from build123d import *

# Parameters (mm, degrees)
SKETCH1_R           = 10
SKETCH1_R_2         = 1
BOSS_EXTRUDE1_DEPTH = 4
SKETCH2_R           = 1.75
SKETCH2_R_2         = 1
BOSS_EXTRUDE2_DEPTH = 22
CHAMFER1_SIZE       = 1
SKETCH3_R           = 1
CUT_EXTRUDE1_DEPTH  = 26.943448113


with BuildPart() as part:
    # Sketch1 → Boss-Extrude1 (new body)
    with BuildSketch(Plane.XY):
        Circle(SKETCH1_R)
        Circle(SKETCH1_R_2, mode=Mode.SUBTRACT)
    extrude(amount=BOSS_EXTRUDE1_DEPTH)

    # Sketch2 → Boss-Extrude2 (add)
    with BuildSketch(Plane.XY.offset(4)):
        Circle(SKETCH2_R)
        Circle(SKETCH2_R_2, mode=Mode.SUBTRACT)
    extrude(amount=BOSS_EXTRUDE2_DEPTH)

    # Chamfer1
    # the kernel refuses this chamfer: 1 mm, written as the material it takes off along each edge
    with BuildSketch(Plane(origin=(0, 0, 26), x_dir=(1, 0, 0), z_dir=(0, -1, 0))) as chamfer1_piece_1:
        Polygon((1.75, -CHAMFER1_SIZE), (1.75 - CHAMFER1_SIZE, 0), (1.75, 0), align=None)
    revolve(axis=Axis((0, 0, 26), (0, 0, 1)), mode=Mode.SUBTRACT)

    # Sketch3 → Cut-Extrude1 (cut, through all)
    with BuildSketch(Plane.XY.offset(4)):
        with Locations((0, 7.5)):
            Circle(SKETCH3_R)
        with Locations((-7.5, 0)):
            Circle(SKETCH3_R)
        with Locations((7.5, 0)):
            Circle(SKETCH3_R)
        with Locations((0, -7.5)):
            Circle(SKETCH3_R)
    extrude(amount=-CUT_EXTRUDE1_DEPTH, mode=Mode.SUBTRACT)


solid = part.part
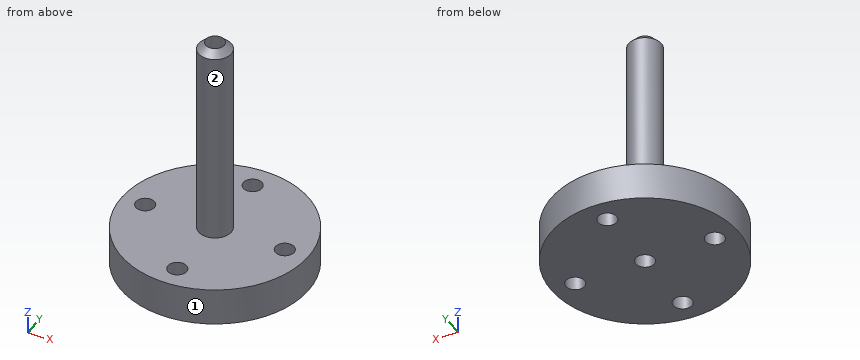
The model under review builds one solid part; all positions refer to its coordinate system, in mm. Face numbers are marked on the shaded views. A direction names the side the tool comes from. Round coordinates to 2 decimals unless told otherwise and drop trailing zeros. Loops run counter-clockwise (first coordinate to the right, second up) from the corner with the lowest first, then second, coordinate; pieces in that order, holes last. Notation, with made-up numbers: M 54,71 L 72,71 A12 cw 72,93 Z; hole C 79.25,19 d7. An arc over 180 degrees is marked long. Answer as CSV lines item,"result". Start each with the question number.
Item 1: For the marked faces 1 and 2, list the 3-axis set-ups (+Z, -Z, +X, -X, +Y, -Y) from which the entire face can be reached by the end or side of a thin tool; tool diameter is ignored.
Item 2: Wall thickness on line 1 (Y direction, x = 0, z = 3.2); line 2 (Y direction, x = 0, z = 14); line 3 (Z direction, x = 0.75, y = 6): over which ranges is each line inside the solid? List them lowest first. Write a range as [from, to].
Item 3: Consider section C-C (y = -7.5). Write out the cut boundary in (x, z), then the cut area to 3 significant figures.
Item 4: Insertion check: P1, Ø1.2, axis at x = 7.5, y = 0, coming from the +Z side; P2, Ø12, axis at x = 2, y = 2.5, coming from the -Z side; P3, Ø3, axis at x = -6, z = 4, coming from the -Y side; P4, Ø6, axis at x = -3, y = -3.5, coming from the +Z side. Each pin has a flat end and moves straight along its axis. Give the tip position at first contact, or say it passes through.
Item 5: Consider section A-A (x = 0). Write out the cut boundary in (y, z).
Answer:
1,face 1,"+Z, -Z"
1,face 2,"+Z"
2,line 1,"y = [-10, -8.5], [-6.5, -1], [1, 6.5], [8.5, 10]"
2,line 2,"y = [-1.75, -1], [1, 1.75]"
2,line 3,"z = [0, 4]"
3,outline,"M -6.61,0 L -1,0 L -1,4 L -6.61,4 Z; M 1,0 L 6.61,0 L 6.61,4 L 1,4 Z"
3,area,"44.9 mm^2"
4,P1,"passes through"
4,P2,"stops at z = 0"
4,P3,"stops at y = -8.93"
4,P4,"stops at z = 25.14"
5,outline,"M -10,0 L -8.5,0 L -8.5,4 L -10,4 Z; M -6.5,0 L -1,0 L -1,25.75 L -1.75,25 L -1.75,4 L -6.5,4 Z; M 1,0 L 6.5,0 L 6.5,4 L 1.75,4 L 1.75,25 L 1,25.75 Z; M 8.5,0 L 10,0 L 10,4 L 8.5,4 Z"
